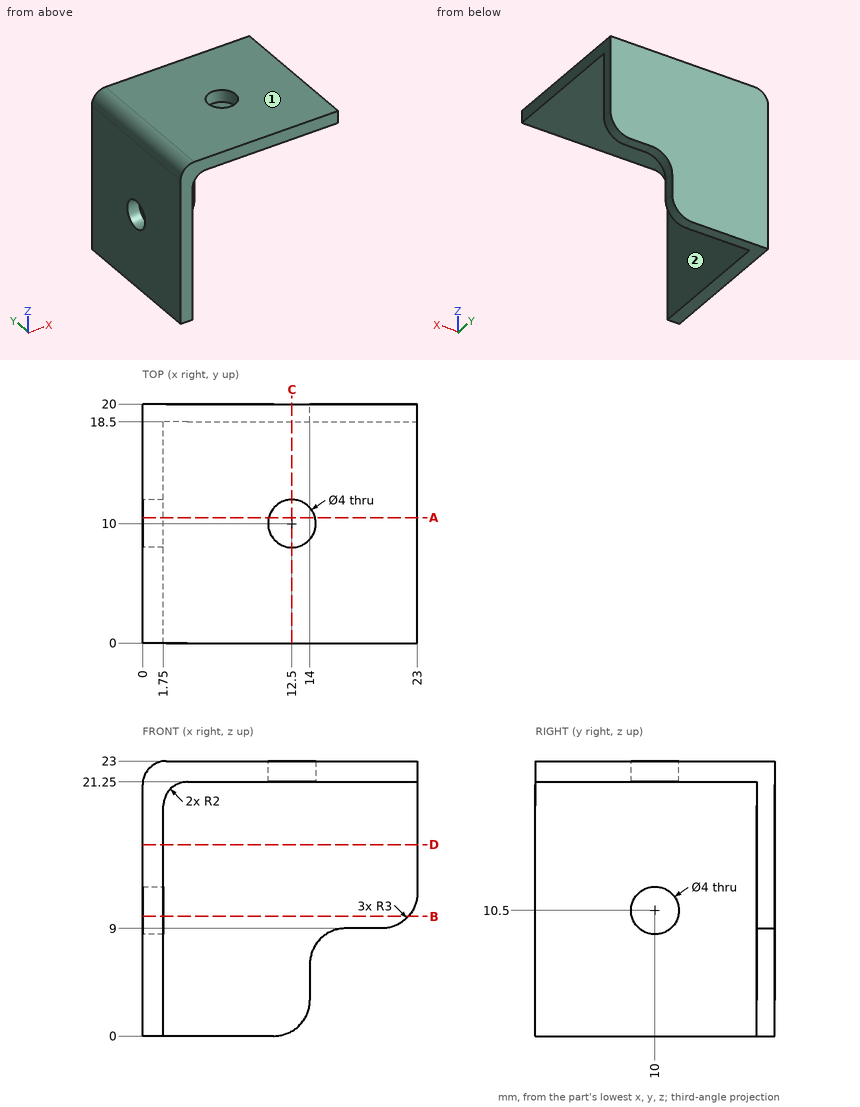
Part print with two shaded views. Sizes in mm from the minimum x, y, z corner. A direction names the side the tool comes from. Round coordinates to 2 decimals unless told otherwise and drop trailing zeros. Write each loop counter-clockwise with the first axis right and the second up, starting at its lowest first coordinate (ties: lowest second). Pieces come first, ordered by that corner, then holes. Notation, with made-up numbers: (26, 39.5) - (75, 39.5) arc R25 cw to (75, 59.5) - close; hole circle Ø11 at (-34, 30). An arc over 180 degrees is marked (long way). Use CSV: the item, a comma, the result in double quotes.
Item 1: Slice it at C-C, the plane x = 12.5. Write the cut outline in (y, z), then the cut area to 3 significant figures.
Results list:
outline,"(0, 21.25) - (8, 21.25) - (8, 23) - (0, 23) - close; (12, 21.25) - (18.5, 21.25) - (18.5, 0.4) - (20, 0.4) - (20, 23) - (12, 23) - close"
area,"59.3 mm²"
Item 2: Slice it at A-A, the plane y = 10.5. Write the cut outline in (x, z), then the cut area to 3 significant figures.
Results list:
outline,"(0, 0) - (1.75, 0) - (1.75, 8.56) - (0, 8.56) - close; (0, 12.44) - (1.75, 12.44) - (1.75, 19.25) arc R2 cw to (3.75, 21.25) - (10.56, 21.25) - (10.56, 23) - (2, 23) arc R2 ccw to (0, 21) - close; (14.44, 21.25) - (23, 21.25) - (23, 23) - (14.44, 23) - close"
area,"63.9 mm²"
Item 3: Tool access for the marked faces 1 and 2: list every direction of +Z, -Z, +X, -X, +Y, -Y with a clear straight run to the whole face (end or side of a thin tool).
Results list:
face 1,"+Z, +X, -X, +Y, -Y"
face 2,"-Z, +X, -Y"
Item 4: Wall check: L1, parallel to Y at x = 12.5, z = 21.9; L2, parallel to X at y = 14, z = 17.75; L3, parallel to Y at x = 13, z = 1.75. Give the ranges that are in metal, low to high.
Results list:
L1,"y = 0 to 8, 12 to 20"
L2,"x = 0 to 1.75"
L3,"y = 18.5 to 20"
Item 5: Slice it at B-B, the plane z = 10. Write the cut outline in (x, y).
Results list:
outline,"(0, 0) - (1.75, 0) - (1.75, 8.06) - (0, 8.06) - close; (0, 11.94) - (1.75, 11.94) - (1.75, 18.5) - (22.24, 18.5) - (22.24, 20) - (0, 20) - close"
Item 6: Slice it at D-D, the plane z = 16. Write the cut outline in (x, y), then the cut area to 3 significant figures.
Results list:
outline,"(0, 0) - (1.75, 0) - (1.75, 18.5) - (23, 18.5) - (23, 20) - (0, 20) - close"
area,"66.9 mm²"
Item 7: Flat gauge pins, fed straight in: P1, Ø2.5, axis at x = 12.5, y = 10, coming from the +Z side; P2, Ø12, axis at x = 9, z = 6.5, coming from the -Y side; P3, Ø0.8, axis at x = 18, y = 19.5, coming from the -Z side; P4, Ø9, axis at x = 9.5, y = 12.5, coming from the -Z side. Where does each tip first touch, or does it go through?
Results list:
P1,"passes through"
P2,"stops at y = 18.5"
P3,"stops at z = 9"
P4,"stops at z = 21.25"
